```python
from build123d import *

# Parameters (mm, degrees)
SALIENTE_EXTRUIR1_DEPTH = 6
CROQUIS7_R              = 40
SALIENTE_EXTRUIR5_DEPTH = 6
SALIENTE_EXTRUIR3_DEPTH = 6
CROQUIS6_R              = 1.75
SALIENTE_EXTRUIR4_DEPTH = 6
CROQUIS8_W              = 6
CROQUIS8_H              = 6
CORTAR_EXTRUIR1_DEPTH   = 25
CROQUIS9_W              = 322
CROQUIS9_H              = 247
CORTAR_EXTRUIR2_DEPTH   = 12
CROQUIS10_R             = 28.25
CORTAR_EXTRUIR3_DEPTH   = 6


with BuildPart() as part:
    # Croquis1 → Saliente-Extruir1 (new body)
    with BuildSketch(Plane(origin=(0, 0, 0), x_dir=(1, 0, 0), z_dir=(0, 1, 0))):
        with BuildLine():
            Line((-161, 103.5), (-38.791887254, 9.756509788))
            ThreePointArc((-38.791887254, 9.756509788), (-40, 0), (-38.791887254, -9.756509788))
            Line((-38.791887254, -9.756509788), (-161, -103.5))
            Line((-161, -103.5), (-161, -123.5))
            Line((-161, -123.5), (-141, -123.5))
            Line((-141, -123.5), (-22.823766962, -32.84928708))
            ThreePointArc((-22.823766962, -32.84928708), (0, -40), (22.823766962, -32.84928708))
            Line((22.823766962, -32.84928708), (141, -123.5))
            Line((141, -123.5), (161, -123.5))
            Line((161, -123.5), (161, -103.5))
            Line((161, -103.5), (38.791887254, -9.756509788))
            ThreePointArc((38.791887254, -9.756509788), (40, 0), (38.791887254, 9.756509788))
            Line((38.791887254, 9.756509788), (161, 103.5))
            Line((161, 103.5), (161, 123.5))
            Line((161, 123.5), (141, 123.5))
            Line((141, 123.5), (22.823766962, 32.84928708))
            ThreePointArc((22.823766962, 32.84928708), (0, 40), (-22.823766962, 32.84928708))
            Line((-22.823766962, 32.84928708), (-141, 123.5))
            Line((-141, 123.5), (-161, 123.5))
            Line((-161, 123.5), (-161, 103.5))
        make_face()
    extrude(amount=SALIENTE_EXTRUIR1_DEPTH)

    # Croquis7 → Saliente-Extruir5 (add)
    with BuildSketch(Plane(origin=(0, 0, 0), x_dir=(-1, 0, 0), z_dir=(0, -1, 0))):
        Circle(CROQUIS7_R)
    extrude(amount=SALIENTE_EXTRUIR5_DEPTH)

    # Croquis5 → Saliente-Extruir3 (add)
    with BuildSketch(Plane.XZ.offset(6)):
        with BuildLine():
            Line((18.896097481, -21), (-18.896097481, -21))
            ThreePointArc((-18.896097481, -21), (-28.25, 0), (-18.896097481, 21))
            Line((-18.896097481, 21), (-13.25, 21))
            Line((-13.25, 21), (-13.25, -11))
            Line((-13.25, -11), (13.25, -11))
            Line((13.25, -11), (13.25, 21))
            Line((13.25, 21), (18.896097481, 21))
            ThreePointArc((18.896097481, 21), (28.25, 0), (18.896097481, -21))
        make_face()
    extrude(amount=SALIENTE_EXTRUIR3_DEPTH)

    # Croquis6 → Saliente-Extruir4 (add)
    with BuildSketch(Plane.XZ.offset(12)):
        with BuildLine():
            Line((-18.896097481, 21), (-13.25, 21))
            Line((-13.25, 21), (-13.25, 3.5))
            ThreePointArc((-13.25, 3.5), (-13.103553391, 3.146446609), (-12.75, 3))
            Line((-12.75, 3), (12.75, 3))
            ThreePointArc((12.75, 3), (13.103553391, 3.146446609), (13.25, 3.5))
            Line((13.25, 3.5), (13.25, 21))
            Line((13.25, 21), (18.896097481, 21))
            ThreePointArc((18.896097481, 21), (28.25, 0), (18.896097481, -21))
            Line((18.896097481, -21), (-18.896097481, -21))
            ThreePointArc((-18.896097481, -21), (-28.25, 0), (-18.896097481, 21))
        make_face()
        with Locations((-8, -5.75)):
            Circle(CROQUIS6_R, mode=Mode.SUBTRACT)
        with Locations((8, -5.75)):
            Circle(CROQUIS6_R, mode=Mode.SUBTRACT)
    extrude(amount=SALIENTE_EXTRUIR4_DEPTH)

    # Croquis8 → Cortar-Extruir1 (cut, through all)
    with BuildSketch(Plane.XZ.offset(18)):
        with Locations((-20, 0)):
            Rectangle(CROQUIS8_W, CROQUIS8_H)
        with Locations((20, 0)):
            Rectangle(CROQUIS8_W, CROQUIS8_H)
    extrude(amount=-CORTAR_EXTRUIR1_DEPTH, mode=Mode.SUBTRACT)

    # Croquis9 → Cortar-Extruir2 (cut)
    with BuildSketch(Plane(origin=(0, 6, 0), x_dir=(1, 0, 0), z_dir=(0, 1, 0))):
        Rectangle(CROQUIS9_W, CROQUIS9_H)
    extrude(amount=-CORTAR_EXTRUIR2_DEPTH, mode=Mode.SUBTRACT)

    # Croquis10 → Cortar-Extruir3 (cut)
    with BuildSketch(Plane(origin=(0, -6, 0), x_dir=(1, 0, 0), z_dir=(0, 1, 0))):
        Circle(CROQUIS10_R)
    extrude(amount=-CORTAR_EXTRUIR3_DEPTH, mode=Mode.SUBTRACT)


solid = part.part
```
Verification items for the finished model (mm, model axes). A direction names the side the tool comes from. Coordinates: 2 decimals unless noted, no trailing zeros. Order: outer loops, then holes, each group sorted by start corner. A loop starts at its lowest first (then second) coordinate and runs counter-clockwise, first axis right, second up. Notation, with made-up numbers: (32.25, 0.25) - (83.25, 0.25) arc R17 cw to (83.25, 23.25) - close; hole circle Ø6 at (-8.5, 81.25). An arc over 180 degrees is marked (long way). Return JSON: item names as keys, results as strings.
(1) Section check D-D, the plane z = 14. Record the cut outline in (x, y), and give its area (3 significant figures).
Filled sheet:
{"outline": "(-24.54, -18) - (-13.25, -18) - (-13.25, -12) - (-24.54, -12) - close; (13.25, -18) - (24.54, -18) - (24.54, -12) - (13.25, -12) - close", "area": "135 mm^2"}
(2) Section check C-C, the plane z = 1.5. Record the cut outline in (x, y).
Filled sheet:
{"outline": "(-28.21, -18) - (-23, -18) - (-23, -12) - (-28.21, -12) - close; (-17, -18) - (17, -18) - (17, -12) - (-17, -12) - close; (23, -18) - (28.21, -18) - (28.21, -12) - (23, -12) - close"}
(3) Access from +Z, -Z, +X, -X, +Y, -Y to the whole of each face (thin tool, end or side, straight path). Record for faces 1 (the flat face through (13.25, -15, 12)), 2 (the flat face through (16, -15, 21)), 3 (the flat face through (20, -15, -3)).
Filled sheet:
{"face 1": "+Z, +Y, -Y", "face 2": "+Z, +X, -X, +Y, -Y", "face 3": "+Y, -Y"}
(4) Mould release check, pull along Z, two halves, no side actions. Record for faces 4 (the cylindrical face through (-28.25, -14.96, -0.33)), 5 (the flat face through (23, -15, 0)), 6 (the flat face through (-16, -15, 21)): pulls with the +Z half, pulls with the -Z half, needs draft (parallel to the pull), parting line crosses it, or undercut.
Filled sheet:
{"face 4": "parting line crosses it", "face 5": "undercut", "face 6": "pulls with the +Z half"}
(5) Thickness scan on line 1 along Z through (x, y) = (8, -15.5); line 2 along X through (y, z) = (-13.45, -2); line 3 along Z through (x, y) = (-9, -14.7). Record the ranges inside material, lowest first.
Filled sheet:
{"line 1": "z = -21 to -7.5, -4 to 3", "line 2": "x = -28.18 to -23, -17 to 17, 23 to 28.18", "line 3": "z = -21 to -7.19, -4.31 to 3"}
(6) Go/stop test with a flat-tipped pin: pin 1 (3 mm diameter, centred on y = -14.5, z = 10.5, fed in from -X). Record where the tip stops, or that it passes through.
Filled sheet:
{"pin 1": "stops at x = -26.78"}
(7) Section check B-B, the plane y = -15.95. Record the cut outline in (x, z), and give its area (3 significant figures).
Filled sheet:
{"outline": "(-18.9, -21) - (18.9, -21) arc R28.25 ccw to (18.9, 21) - (13.25, 21) - (13.25, 3.5) arc R0.5 cw to (12.75, 3) - (-12.75, 3) arc R0.5 cw to (-13.25, 3.5) - (-13.25, 21) - (-18.9, 21) arc R28.25 ccw to start; hole (-23, -3) - (-17, -3) - (-17, 3) - (-23, 3) - close; hole circle Ø3.5 at (-8, -5.75); hole circle Ø3.5 at (8, -5.75); hole (17, -3) - (23, -3) - (23, 3) - (17, 3) - close", "area": "1,560 mm^2"}
(8) Section check A-A, the plane x = -21. Record the cut outline in (y, z).
Filled sheet:
{"outline": "(-18, -18.9) - (-12, -18.9) - (-12, -3) - (-18, -3) - close; (-18, 3) - (-12, 3) - (-12, 18.9) - (-18, 18.9) - close"}
